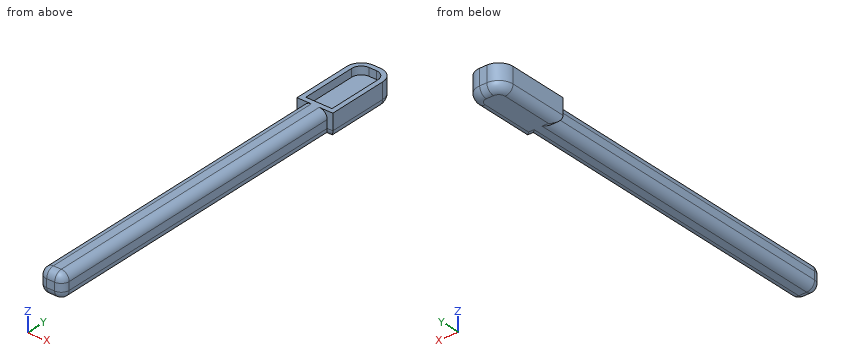
```python
from build123d import *

# Parameters (mm, degrees)
EXTRUDE_1_DEPTH     = 3
CUT_EXTRUDE_1_DEPTH = 1
FILLET_3_R          = 1


with BuildPart() as part:
    # 草图1 → 凸台-拉伸1 (new body)
    with BuildSketch(Plane.XY):
        with BuildLine():
            Line((3, 40), (3.703089902, 40))
            Line((3.703089902, 40), (3.703089902, 47.546153846))
            ThreePointArc((3.703089902, 47.546153846), (3.175882108, 48.818946052), (1.903089902, 49.346153846))
            Line((1.903089902, 49.346153846), (1.003089902, 49.346153846))
            ThreePointArc((1.003089902, 49.346153846), (-0.269702304, 48.818946052), (-0.796910098, 47.546153846))
            Line((-0.796910098, 47.546153846), (-0.796910098, 40))
            Line((-0.796910098, 40), (0, 40))
            Line((0, 40), (0, 0))
            Line((0, 0), (3, 0))
            Line((3, 0), (3, 40))
        make_face()
    extrude(amount=EXTRUDE_1_DEPTH)

    # 草图2 → 切除-拉伸1 (cut)
    with BuildSketch(Plane.XY.offset(3)):
        with BuildLine():
            Line((3.103089902, 40.6), (3.103089902, 47.546153846))
            ThreePointArc((3.103089902, 47.546153846), (2.751618039, 48.394681984), (1.903089902, 48.746153846))
            Line((1.903089902, 48.746153846), (1.003089902, 48.746153846))
            ThreePointArc((1.003089902, 48.746153846), (0.154561764, 48.394681984), (-0.196910098, 47.546153846))
            Line((-0.196910098, 47.546153846), (-0.196910098, 40.6))
            Line((-0.196910098, 40.6), (3.103089902, 40.6))
        make_face()
    extrude(amount=-CUT_EXTRUDE_1_DEPTH, mode=Mode.SUBTRACT)

    # 圆角3
    fillet_3_edges = [part.edges().sort_by_distance(p)[0] for p in [
        (3, 20, 3),
        (-0.269702304, 48.818946052, 0),
        (1.453089902, 49.346153846, 0),
        (3.175882108, 48.818946052, 0),
        (3.703089902, 43.773076923, 0),
        (3.351544951, 40, 0),
        (3, 20, 0),
        (1.5, 0, 0),
        (0, 20, 0),
        (3, 0, 1.5),
        (0, 0, 1.5),
        (0, 20, 3),
        (1.5, 0, 3),
        (-0.398455049, 40, 0),
        (-0.796910098, 43.773076923, 0),
    ]]
    fillet(fillet_3_edges, radius=FILLET_3_R)


solid = part.part
```
The listing builds one solid part. Answer for the finished solid, in the listing's coordinates (mm). Coordinates: 2 decimals unless noted, no trailing zeros. Write each loop counter-clockwise with the first axis right and the second up, starting at its lowest first coordinate (ties: lowest second). Pieces come first, ordered by that corner, then holes. Notation, with made-up numbers: (47.25, 68) - (84.25, 68) arc R22 cw to (84.25, 78) - close; hole circle Ø2 at (87, 63.25). An arc over 180 degrees is marked (long way). Return JSON: item names as keys, results as strings. Group by question number.
1. A cutting plane is placed at A-A, the plane y = 24.5. Determine the outline of the cut face in (x, z), plus the area to 3 significant figures.
2. Straight lines are drawn through the part: L1, parallel to X at y = 31, z = 1.15; L2, parallel to Y at x = 1, z = 2.45; L3, parallel to Y at x = -0.45, z = 2.1. For each, find the intervals that lie inside material, in ascending order.
3. A cutting plane is placed at B-B, the plane z = 1.6. Determine the outline of the cut face in (x, y), plus the area to 3 significant figures.
4. A cutting plane is placed at C-C, the plane y = 44. Determine the outline of the cut face in (x, z), plus the area to 3 significant figures.
5. Given pin 1 (0.7 mm diameter, centred on x = 1.5, z = 2.5, fed in from -Y); pin 2 (1 mm diameter, centred on x = 0, z = 2, fed in from -Y); pin 3 (0.5 mm diameter, centred on y = 14, z = 1.5, fed in from +X), each flat-ended and moving along its own axis, determine where each tip first touches the part or whether it passes through.
Ans:
{
 "1": {"outline": "(0, 1) arc R1 ccw to (1, 0) - (2, 0) arc R1 ccw to (3, 1) - (3, 2) arc R1 ccw to (2, 3) - (1, 3) arc R1 ccw to (0, 2) - close", "area": "8.14 mm²"},
 "2": {"L1": "0 to 3", "L2": "0.11 to 40.6, 48.75 to 49.35", "L3": "40 to 48.61"},
 "3": {"outline": "(-0.8, 40) - (0, 40) - (0, 1) arc R1 ccw to (1, 0) - (2, 0) arc R1 ccw to (3, 1) - (3, 40) - (3.7, 40) - (3.7, 47.55) arc R1.8 ccw to (1.9, 49.35) - (1, 49.35) arc R1.8 ccw to (-0.8, 47.55) - close", "area": "160 mm²"},
 "4": {"outline": "(-0.8, 1) arc R1 ccw to (0.2, 0) - (2.7, 0) arc R1 ccw to (3.7, 1) - (3.7, 3) - (3.1, 3) - (3.1, 2) - (-0.2, 2) - (-0.2, 3) - (-0.8, 3) - close", "area": "9.77 mm²"},
 "5": {"pin 1": "y = 0.01", "pin 2": "y = 0.13", "pin 3": "x = 3"}
}
